```python
from build123d import *

# Parameters (mm, degrees)
BOX001_W     = 74
BOX001_H     = 13
BOX001_DEPTH = 14
FILLET007_R  = 5
FILLET008_R  = 5
BOX_W        = 78
BOX_H        = 13
BOX_DEPTH    = 16
FILLET_R     = 5
FILLET006_R  = 5


with BuildPart() as fillet008:
    # Box001 → Box001 (new body)
    with BuildSketch(Plane(origin=(-65, 17, -11.5), x_dir=(1, 0, 0), z_dir=(0, 0, 1))):
        with Locations((37, 6.5)):
            Rectangle(BOX001_W, BOX001_H)
    extrude(amount=BOX001_DEPTH)

    # Fillet007
    fillet007_edges = [fillet008.edges().sort_by_distance(p)[0] for p in [
        (9, 30, -4.5),
    ]]
    fillet(fillet007_edges, radius=FILLET007_R)

    # Fillet008
    fillet008_edges = [fillet008.edges().sort_by_distance(p)[0] for p in [
        (-65, 30, -4.5),
    ]]
    fillet(fillet008_edges, radius=FILLET008_R)


with BuildPart() as fillet008_1:
    # Fillet008 placement: moved
    add(fillet008.part.moved(Location((2, -2, 1))))


with BuildPart() as i2c_hosting:
    # Box → Box (new body)
    with BuildSketch(Plane(origin=(-65, 17, -13.5), x_dir=(1, 0, 0), z_dir=(0, 0, 1))):
        with Locations((39, 6.5)):
            Rectangle(BOX_W, BOX_H)
    extrude(amount=BOX_DEPTH)

    # Fillet
    fillet_edges = [i2c_hosting.edges().sort_by_distance(p)[0] for p in [
        (13, 30, -5.5),
    ]]
    fillet(fillet_edges, radius=FILLET_R)

    # Fillet006
    fillet006_edges = [i2c_hosting.edges().sort_by_distance(p)[0] for p in [
        (-65, 30, -5.5),
    ]]
    fillet(fillet006_edges, radius=FILLET006_R)

    # Cut: cut Fillet008
    add(fillet008_1.part, mode=Mode.SUBTRACT)


with BuildPart() as i2c_hosting_1:
    # Cut placement: moved
    add(i2c_hosting.part.moved(Location((-1.54, 0, 4.2))))


solid = i2c_hosting_1.part
```
Read the model definition and answer for the solid it produces. Units are mm, in the model's axes. A direction names the side the tool comes from. Give positions to 0.01 mm unless a question says otherwise; leave off trailing zeros. Loops run counter-clockwise (first coordinate to the right, second up) from the corner with the lowest first, then second, coordinate; pieces in that order, holes last.
Item 1: The mould has two halves that part along X. Classify faces 3 (the flat face through (-64.54, 20, 0)), 4 (the flat face through (11.46, 21, -1)), 5 (the flat face through (-28, 29, 6.7)): released by +X, released by -X, zero draft, split by the parting line, or undercut.
Item 2: The part is cut by section D-D (y = 26.25). Write down the section's boundary in (x, z).
Item 3: The part is cut by section A-A (z = 1.25). Write down the section's boundary in (x, y), and give its area (3 significant figures).
Item 4: For faces 1 (the cylindrical face through (-63.04, 26.57, 0.29)), 2 (the flat face through (-28, 24, -9.3)), determine the directions among +Z, -Z, +X, -X, +Y, -Y from which every point of the face is accessible in a straight line to the end or side of a thin tool.
Item 5: This flat-tipped pin is pushed along its axis until it touches: pin 1 Ø3.5 at (x, y) = (-21, 21) entering from +Z. Where does it stop, or does it pass through?
Item 6: The part is cut by section C-C (x = -13). Write down the section's boundary in (y, z).
Item 7: Find the intervals of material crossed by line 1 along Z through (x, y) = (-32, 26.5); line 2 along X through (y, z) = (19.25, 2.5); line 3 along Y through (x, z) = (-34, -0.25), in increasing order.
Item 8: The part is cut by section B-B (y = 22). Write down the section's boundary in (x, z).
Taken from the geometry:
1. face 3: undercut
1. face 4: released by +X
1. face 5: zero draft
2. outline: (-66.38, -9.3) - (11.3, -9.3) - (11.3, 6.7) - (8.26, 6.7) - (8.26, -6.3) - (-63.34, -6.3) - (-63.34, 6.7) - (-66.38, 6.7) - close
3. outline: (-66.54, 17) - (-64.54, 17) - (-64.54, 23) arc R5 cw to (-59.54, 28) - (4.46, 28) arc R5 cw to (9.46, 23) - (9.46, 17) - (11.46, 17) - (11.46, 25) arc R5 ccw to (6.46, 30) - (-61.54, 30) arc R5 ccw to (-66.54, 25) - close
3. area: 200 mm2
4. face 1: +Z, -Y
4. face 2: -Z, +X, -X, +Y, -Y
5. pin 1: stops at z = -6.3
6. outline: (17, -9.3) - (30, -9.3) - (30, 6.7) - (28, 6.7) - (28, -6.3) - (17, -6.3) - close
7. line 1: z = -9.3 to -6.3
7. line 2: x = -66.54 to -64.54, 9.46 to 11.46
7. line 3: y = 28 to 30
8. outline: (-66.54, -9.3) - (11.46, -9.3) - (11.46, 6.7) - (9.46, 6.7) - (9.46, -6.3) - (-64.54, -6.3) - (-64.54, 6.7) - (-66.54, 6.7) - close
